The drawing under review shows one solid part. Ordinate dimensions are in mm from its lowest x, y, z. A direction names the side the tool comes from. Coordinates: 2 decimals unless noted, no trailing zeros. Loops run counter-clockwise (first coordinate to the right, second up) from the corner with the lowest first, then second, coordinate; pieces in that order, holes last.
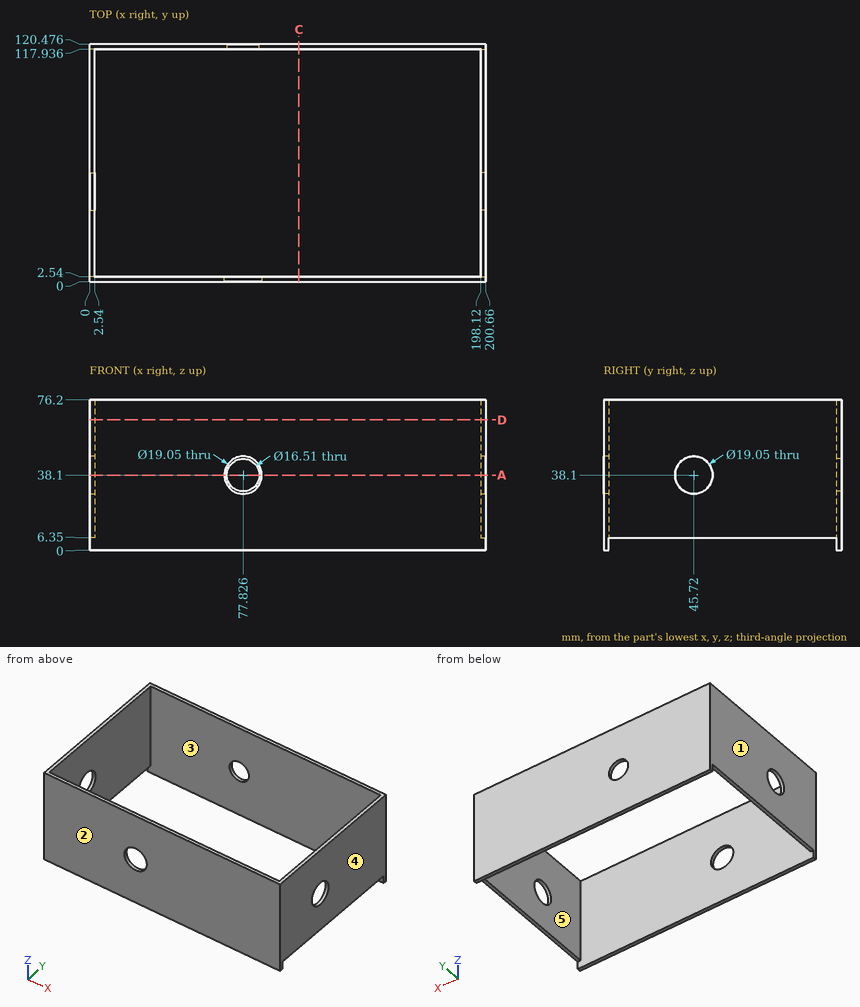
Q1. Take a section at D-D, the plane z = 66. Write out the cut boundary in (x, y).
Q2. Take a section at A-A, the plane z = 38.1. Give the number of separate pieces and of enclosed holes in the cut face, then the cut area to 3 significant figures.
Q3. The part is to be moulded in two halves that separate along X. For the marked faces 1, 2 and 3, say which applies: pulls with the +X half, pulls with the -X half, needs draft (parallel to the pull), parting line crosses it, or undercut.
Q4. Machinability: for the marked faces 4 and 5, which of the approach directions +Z, -Z, +X, -X, +Y, -Y give a long, thin tool a straight path to every point of the face, cutting with its end or side? Answer none if there is none.
Q5. Clearance check with flat-ended pins moving along their axes: pin 1 Ø0.8 at (x, y) = (1.5, 37) entering from -Z; pin 2 Ø17 at (y, z) = (45.72, 38.1) entering from +X. State where each tip first meets the part, or that it passes through.
Q6. For line 1 (Y direction, x = 1, z = 38) (1 decimal); line 2 (Y direction, x = 30, z = 69); line 3 (X direction, y = 99, z = 64), list the stretches that pass through material, from the lowest coordinate up.
Q7. Take a section at C-C, the plane x = 106. Write out the cut boundary in (y, z).
Entries:
1. outline: (0, 0) - (200.66, 0) - (200.66, 120.48) - (0, 120.48) - close; hole (2.54, 2.54) - (198.12, 2.54) - (198.12, 117.94) - (2.54, 117.94) - close
2. separate pieces: 4
2. enclosed holes: 0
2. area: 1,420 mm2
3. face 1: pulls with the -X half
3. face 2: needs draft
3. face 3: undercut
4. face 4: +Z, -Z, +X, +Y, -Y
4. face 5: +Z, -Z
5. pin 1: stops at z = 6.35
5. pin 2: passes through
6. line 1: y = 0 to 36.2, 55.2 to 120.5
6. line 2: y = 0 to 2.54, 117.94 to 120.48
6. line 3: x = 0 to 2.54, 198.12 to 200.66
7. outline: (0, 0) - (2.54, 0) - (2.54, 76.2) - (0, 76.2) - close; (117.94, 0) - (120.48, 0) - (120.48, 76.2) - (117.94, 76.2) - close
